Can you work these out from the model? Positions are in its coordinate system, mm. A direction names the side the tool comes from. Round coordinates to 2 decimals unless told otherwise and drop trailing zeros. Order: outer loops, then holes, each group sorted by start corner. A loop starts at its lowest first (then second) coordinate and runs counter-clockwise, first axis right, second up.
Q1. If we section it at A-A (x = 32.5): Please give me the cut outline in (y, z).
Q2. We'd pull the mould along Y, two halves only. Please class faces 3 (the face through (32, 35.306, 1)), 4 (the face through (28.446, 19.973, 1.417)), 5 (the face through (25, 16, 2.794)): pulls with the +Y half, pulls with the -Y half, needs draft (parallel to the pull), parting line crosses it, or undercut.
Q3. For faces 1 (the face through (32, 0, -17)), 2 (the face through (32, -1, -35.306)), which set-ups out of +Z, -Z, +X, -X, +Y, -Y let a thin tool reach every point of the face, with its end or its side?
Q4. If we section it at D-D (z = -29.5): Please give me the cut outline in (x, y), plus the area to 3 significant figures.
Q5. If I drill on line 1 (Y direction, x = 32.5, z = 1.1); line 2 (Z direction, x = 54, y = 22.5); line 3 (Y direction, x = 60.5, z = -3.5), over which ranges is the centre line in solid material (lowest first)?
Q6. Will these pins go through, and if not, where does the flat tip stop? P1, Ø10.5, axis at x = 42.5, y = 12.5, coming from the -Z side; P2, Ø8, axis at x = 12.5, z = -23.5, coming from the +Y side.
Q7. If we section it at C-C (x = 58): Please give me the cut outline in (y, z).
Q8. If we section it at B-B (y = 12): Please give me the cut outline in (x, z), plus the area to 3 significant figures.
from build123d import *

# Parameters (mm, degrees)
BOSS_EXTRUDE1_DEPTH = 65
SKETCH2_R           = 5.5
CUT_EXTRUDE1_DEPTH  = 65


with BuildPart() as part:
    # Sketch1 → Boss-Extrude1 (new body)
    with BuildSketch(Plane(origin=(0, 0, 0), x_dir=(0, 0, -1), z_dir=(1, 0, 0))):
        Polygon((0, 35.306), (0, 0), (35.306, 0), (35.306, -2.794), (-2.794, -2.794), (-2.794, 35.306), align=None)
    extrude(amount=BOSS_EXTRUDE1_DEPTH)

    # Sketch2 → Cut-Extrude1 (cut)
    with BuildSketch(Plane.XY.offset(2.794)):
        with Locations((32.5, 16.256)):
            Circle(SKETCH2_R)
    extrude(amount=-CUT_EXTRUDE1_DEPTH, mode=Mode.SUBTRACT)


solid = part.part
Solution:
1. outline: (-2.79, -35.31) - (0, -35.31) - (0, 0) - (10.76, 0) - (10.76, 2.79) - (-2.79, 2.79) - close; (21.76, 0) - (35.31, 0) - (35.31, 2.79) - (21.76, 2.79) - close
2. face 3: pulls with the +Y half
2. face 4: undercut
2. face 5: needs draft
3. face 1: -Z, +X, -X, +Y
3. face 2: -Z, +X, -X, +Y, -Y
4. outline: (0, -2.79) - (65, -2.79) - (65, 0) - (0, 0) - close
4. area: 182 mm2
5. line 1: y = -2.79 to 10.76, 21.76 to 35.31
5. line 2: z = 0 to 2.79
5. line 3: y = -2.79 to 0
6. P1: stops at z = 0
6. P2: stops at y = 0
7. outline: (-2.79, -35.31) - (0, -35.31) - (0, 0) - (35.31, 0) - (35.31, 2.79) - (-2.79, 2.79) - close
8. outline: (0, 0) - (29.02, 0) - (29.02, 2.79) - (0, 2.79) - close; (35.98, 0) - (65, 0) - (65, 2.79) - (35.98, 2.79) - close
8. area: 162 mm2
